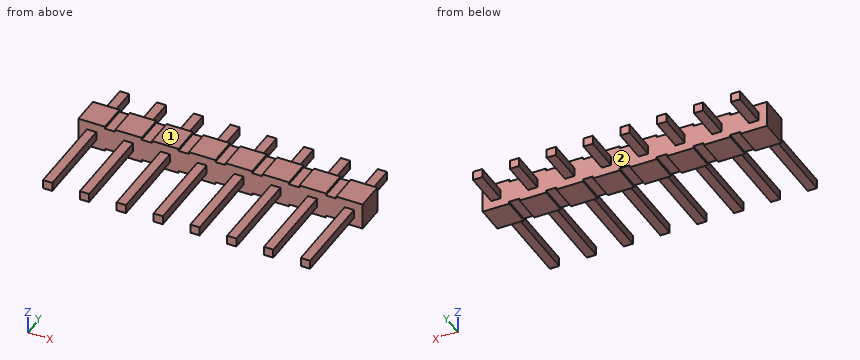
from build123d import *

# Parameters (mm, degrees)
SKETCH1_W                = 1.85
SKETCH1_H                = 1.85
SKETCH1_W_2              = 0.65
SKETCH1_H_2              = 0.62
SKETCH1_W_3              = 0.72
SKETCH1_H_3              = 1.55
BOSS_EXTRUDE1_DEPTH      = 2
BOSS_EXTRUDE2_DEPTH      = 4.5
BOSS_EXTRUDE2_DEPTH_BACK = 6
SKETCH1_3_W              = 0.65
SKETCH1_3_H              = 0.62


with BuildPart() as part:
    # Sketch1 → Boss-Extrude1 (new body)
    # profile 1 of 15: a face of its own
    with BuildSketch(Plane(origin=(0, 0, 0), x_dir=(1, 0, 0), z_dir=(0, 1, 0))):
        with Locations((-8.825, 0)):
            Rectangle(SKETCH1_W, SKETCH1_H)
        with Locations((-8.825, 0)):
            Rectangle(SKETCH1_W_2, SKETCH1_H_2, mode=Mode.SUBTRACT)
    # profile 2 of 15: a face of its own
    with BuildSketch(Plane(origin=(0, 0, 0), x_dir=(1, 0, 0), z_dir=(0, 1, 0))):
        with Locations((-7.54, 0)):
            Rectangle(SKETCH1_W_3, SKETCH1_H_3)
    # profile 3 of 15: a face of its own
    with BuildSketch(Plane(origin=(0, 0, 0), x_dir=(1, 0, 0), z_dir=(0, 1, 0))):
        with Locations((-6.255, 0)):
            Rectangle(SKETCH1_W, SKETCH1_H)
        with Locations((-6.255, 0)):
            Rectangle(SKETCH1_W_2, SKETCH1_H_2, mode=Mode.SUBTRACT)
    # profile 4 of 15: a face of its own
    with BuildSketch(Plane(origin=(0, 0, 0), x_dir=(1, 0, 0), z_dir=(0, 1, 0))):
        with Locations((-4.97, 0)):
            Rectangle(SKETCH1_W_3, SKETCH1_H_3)
    # profile 5 of 15: a face of its own
    with BuildSketch(Plane(origin=(0, 0, 0), x_dir=(1, 0, 0), z_dir=(0, 1, 0))):
        with Locations((-3.685, 0)):
            Rectangle(SKETCH1_W, SKETCH1_H)
        with Locations((-3.685, 0)):
            Rectangle(SKETCH1_W_2, SKETCH1_H_2, mode=Mode.SUBTRACT)
    # profile 6 of 15: a face of its own
    with BuildSketch(Plane(origin=(0, 0, 0), x_dir=(1, 0, 0), z_dir=(0, 1, 0))):
        with Locations((-2.4, 0)):
            Rectangle(SKETCH1_W_3, SKETCH1_H_3)
    # profile 7 of 15: a face of its own
    with BuildSketch(Plane(origin=(0, 0, 0), x_dir=(1, 0, 0), z_dir=(0, 1, 0))):
        with Locations((-1.115, 0)):
            Rectangle(SKETCH1_W, SKETCH1_H)
        with Locations((-1.115, 0)):
            Rectangle(SKETCH1_W_2, SKETCH1_H_2, mode=Mode.SUBTRACT)
    # profile 8 of 15: a face of its own
    with BuildSketch(Plane(origin=(0, 0, 0), x_dir=(1, 0, 0), z_dir=(0, 1, 0))):
        with Locations((0.17, 0)):
            Rectangle(SKETCH1_W_3, SKETCH1_H_3)
    # profile 9 of 15: a face of its own
    with BuildSketch(Plane(origin=(0, 0, 0), x_dir=(1, 0, 0), z_dir=(0, 1, 0))):
        with Locations((1.455, 0)):
            Rectangle(SKETCH1_W, SKETCH1_H)
        with Locations((1.455, 0)):
            Rectangle(SKETCH1_W_2, SKETCH1_H_2, mode=Mode.SUBTRACT)
    # profile 10 of 15: a face of its own
    with BuildSketch(Plane(origin=(0, 0, 0), x_dir=(1, 0, 0), z_dir=(0, 1, 0))):
        with Locations((2.74, 0)):
            Rectangle(SKETCH1_W_3, SKETCH1_H_3)
    # profile 11 of 15: a face of its own
    with BuildSketch(Plane(origin=(0, 0, 0), x_dir=(1, 0, 0), z_dir=(0, 1, 0))):
        with Locations((4.025, 0)):
            Rectangle(SKETCH1_W, SKETCH1_H)
        with Locations((4.025, 0)):
            Rectangle(SKETCH1_W_2, SKETCH1_H_2, mode=Mode.SUBTRACT)
    # profile 12 of 15: a face of its own
    with BuildSketch(Plane(origin=(0, 0, 0), x_dir=(1, 0, 0), z_dir=(0, 1, 0))):
        with Locations((5.31, 0)):
            Rectangle(SKETCH1_W_3, SKETCH1_H_3)
    # profile 13 of 15: a face of its own
    with BuildSketch(Plane(origin=(0, 0, 0), x_dir=(1, 0, 0), z_dir=(0, 1, 0))):
        with Locations((6.595, 0)):
            Rectangle(SKETCH1_W, SKETCH1_H)
        with Locations((6.595, 0)):
            Rectangle(SKETCH1_W_2, SKETCH1_H_2, mode=Mode.SUBTRACT)
    # profile 14 of 15: a face of its own
    with BuildSketch(Plane(origin=(0, 0, 0), x_dir=(1, 0, 0), z_dir=(0, 1, 0))):
        with Locations((7.88, 0)):
            Rectangle(SKETCH1_W_3, SKETCH1_H_3)
    # profile 15 of 15: a face of its own
    with BuildSketch(Plane(origin=(0, 0, 0), x_dir=(1, 0, 0), z_dir=(0, 1, 0))):
        with Locations((9.165, 0)):
            Rectangle(SKETCH1_W, SKETCH1_H)
        with Locations((9.165, 0)):
            Rectangle(SKETCH1_W_2, SKETCH1_H_2, mode=Mode.SUBTRACT)
    extrude(amount=BOSS_EXTRUDE1_DEPTH)

    # Sketch1_3 → Boss-Extrude2 (add, two sides: drawn at the far end of the back side and taken through both)
    with BuildSketch(Plane(origin=(0, 0, 0), x_dir=(1, 0, 0), z_dir=(0, 1, 0)).offset(-BOSS_EXTRUDE2_DEPTH_BACK)):
        with Locations((-8.825, 0)):
            Rectangle(SKETCH1_3_W, SKETCH1_3_H)
        with Locations((-6.255, 0)):
            Rectangle(SKETCH1_3_W, SKETCH1_3_H)
        with Locations((-3.685, 0)):
            Rectangle(SKETCH1_3_W, SKETCH1_3_H)
        with Locations((-1.115, 0)):
            Rectangle(SKETCH1_3_W, SKETCH1_3_H)
        with Locations((1.455, 0)):
            Rectangle(SKETCH1_3_W, SKETCH1_3_H)
        with Locations((4.025, 0)):
            Rectangle(SKETCH1_3_W, SKETCH1_3_H)
        with Locations((6.595, 0)):
            Rectangle(SKETCH1_3_W, SKETCH1_3_H)
        with Locations((9.165, 0)):
            Rectangle(SKETCH1_3_W, SKETCH1_3_H)
    extrude(amount=BOSS_EXTRUDE2_DEPTH + BOSS_EXTRUDE2_DEPTH_BACK)


solid = part.part
Can you work these out from the model? Positions are in its coordinate system, mm. Face numbers are marked on the shaded views. Coordinates: 2 decimals unless noted, no trailing zeros. Write each loop counter-clockwise with the first axis right and the second up, starting at its lowest first coordinate (ties: lowest second). Pieces come first, ordered by that corner, then holes.
Q1. For P1, Ø2, axis at x = 3, y = -5, coming from the +Z side; P2, Ø0.5, axis at y = -4, z = 0, coming from the -X side; P3, Ø0.7, axis at y = -2, z = 0, coming from the +X side, each with a flat end and sliding along its axis, tell me the tip position at first contact or that it passes through.
Results found:
P1: stops at z = 0.31
P2: stops at x = -9.15
P3: stops at x = 9.49
Q2. Please list where these lines run through material, in increasing order: L1, parallel to Y at x = -1.75, z = 0.05; L2, parallel to Z at x = -3.5, y = 3.75.
Results found:
L1: y = 0 to 2
L2: z = -0.31 to 0.31
Q3. If we mould it in two halves opening along X, with no side actions, what happens to the marked faces 1 and 2? For each: +X half, -X half, draft (parallel to the pull), parting line (faces both ways), or undercut.
Results found:
face 1: draft
face 2: undercut
Q4. Imagine slicing it at D-D, the plane x = -3. List the corners of the cut face in (y, z) for me (3 decimals), plus the area to 3 significant figures.
Results found:
outline: (0, -0.925) - (2, -0.925) - (2, 0.925) - (0, 0.925) - close
area: 3.70 mm2
Q5. Imagine slicing it at A-A, the plane y = -2. Count the separate pieces of the cut face and the enclosed holes in it, plus the area to 3 significant figures.
Results found:
separate pieces: 8
enclosed holes: 0
area: 3.22 mm2
Q6. Imagine slicing it at C-C, the plane z = 0.55. List the corners of the cut face in (x, y) for me.
Results found:
outline: (-9.75, 0) - (10.09, 0) - (10.09, 2) - (-9.75, 2) - close
Q7. Imagine slicing it at B-B, the plane x = -1. List the corners of the cut face in (y, z) for me (3 decimals), plus the area to 3 significant figures.
Results found:
outline: (-6, -0.31) - (0, -0.31) - (0, -0.925) - (2, -0.925) - (2, -0.31) - (4.5, -0.31) - (4.5, 0.31) - (2, 0.31) - (2, 0.925) - (0, 0.925) - (0, 0.31) - (-6, 0.31) - close
area: 8.97 mm2
